Source: three-view drawing plus pictorial views. Frame: mm from the lowest corner of the part. A direction names the side the tool comes from. Round coordinates to 2 decimals unless told otherwise and drop trailing zeros. Loops run counter-clockwise (first coordinate to the right, second up) from the corner with the lowest first, then second, coordinate; pieces in that order, holes last. Notation, with made-up numbers: M 88,12.25 L 140,12.25 A21 cw 140,22.25 Z; hole C -28.75,40 d1. An arc over 180 degrees is marked long. Write each question's results on one line, items separated by ' | '.
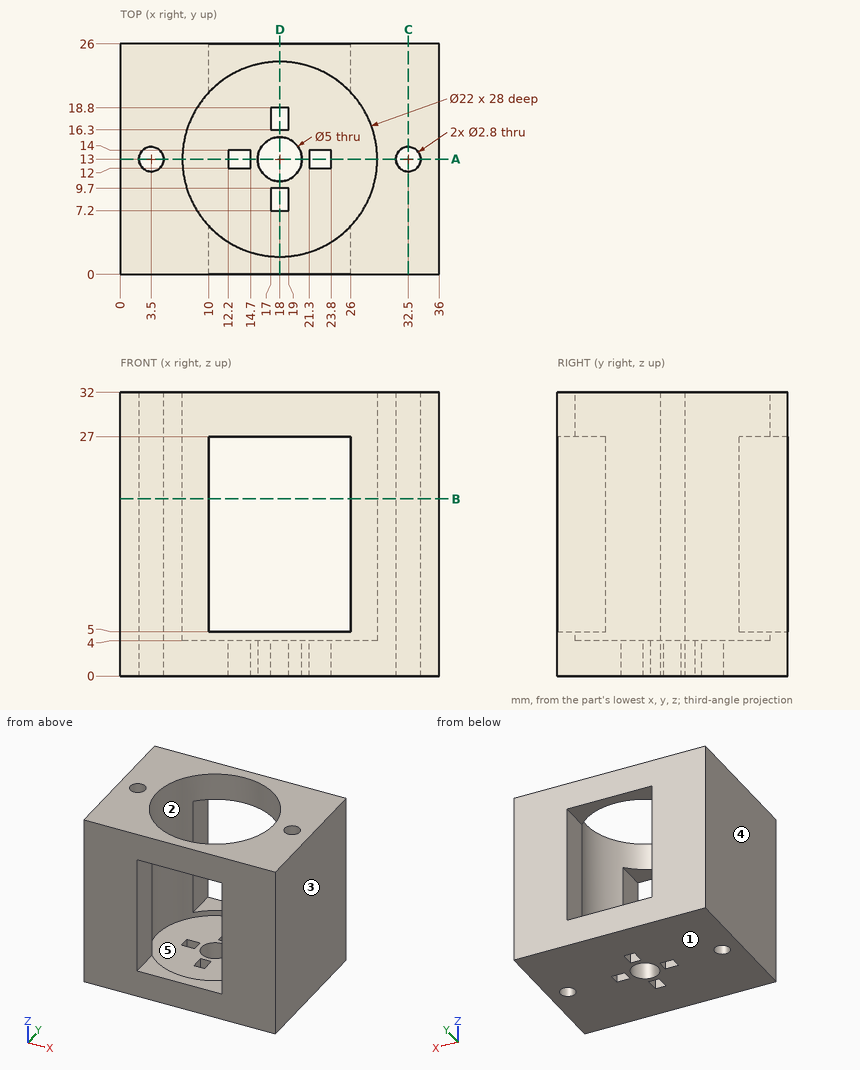
1. Section B-B (z = 20). Output: boundary loops of the cut face in (x, y), then the cut area to 3 significant figures.
Answer key:
outline: M 0,0 L 10,0 L 10,5.45 A11 cw 10,20.55 L 10,26 L 0,26 Z; M 26,0 L 36,0 L 36,26 L 26,26 L 26,20.55 A11 cw 26,5.45 Z; hole C 3.5,13 d2.8; hole C 32.5,13 d2.8 | area: 445 mm²
2. Draft query along X for the marked faces 1, 2 and 3. Return one class per face: pulls with the +X half, pulls with the -X half, needs draft (parallel to the pull), parting line crosses it, or undercut.
Answer key:
face 1: needs draft | face 2: undercut | face 3: pulls with the +X half
3. Pin query (flat end, axial travel): P1, Ø6.5, axis at x = 12.5, y = 10.5, coming from the +Z side; P2, Ø2, axis at x = 32.5, y = 13, coming from the +Z side. Return the tip coordinate at first contact, or that it passes through.
Answer key:
P1: stops at z = 4 | P2: passes through
4. Section A-A (y = 13). Output: boundary loops of the cut face in (x, z).
Answer key:
outline: M 0,0 L 2.1,0 L 2.1,32 L 0,32 Z; M 4.9,0 L 12.2,0 L 12.2,4 L 7,4 L 7,32 L 4.9,32 Z; M 14.7,0 L 15.5,0 L 15.5,4 L 14.7,4 Z; M 20.5,0 L 21.3,0 L 21.3,4 L 20.5,4 Z; M 23.8,0 L 31.1,0 L 31.1,32 L 29,32 L 29,4 L 23.8,4 Z; M 33.9,0 L 36,0 L 36,32 L 33.9,32 Z
5. Section D-D (x = 18). Output: boundary loops of the cut face in (y, z).
Answer key:
outline: M 0,0 L 7.2,0 L 7.2,4 L 2,4 L 2,5 L 0,5 Z; M 0,27 L 2,27 L 2,32 L 0,32 Z; M 9.7,0 L 10.5,0 L 10.5,4 L 9.7,4 Z; M 15.5,0 L 16.3,0 L 16.3,4 L 15.5,4 Z; M 18.8,0 L 26,0 L 26,5 L 24,5 L 24,4 L 18.8,4 Z; M 24,27 L 26,27 L 26,32 L 24,32 Z
6. Ray query, probe 1 along Y at (x, z) = (18, 3.05); probe 2 along X at (y, z) = (21.75, 21.5); probe 3 along X at (y, z) = (13, 1.45). Return the intervals inside material, ascending.
Answer key:
probe 1: y = 0 to 7.2, 9.7 to 10.5, 15.5 to 16.3, 18.8 to 26 | probe 2: x = 0 to 10, 26 to 36 | probe 3: x = 0 to 2.1, 4.9 to 12.2, 14.7 to 15.5, 20.5 to 21.3, 23.8 to 31.1, 33.9 to 36
7. Access query for the marked faces 4 and 5. Directions: +Z, -Z, +X, -X, +Y, -Y. A direction counts if a zero-diameter tool reaches every point of the face in a straight line with its end or side. Return the directions, or none.
Answer key:
face 4: +Z, -Z, -X, +Y, -Y | face 5: +Z
8. Section C-C (x = 32.5). Output: boundary loops of the cut face in (y, z).
Answer key:
outline: M 0,0 L 11.6,0 L 11.6,32 L 0,32 Z; M 14.4,0 L 26,0 L 26,32 L 14.4,32 Z
